from build123d import *

# Parameters (mm, degrees)
F0_R     = 3.5
F1_DEPTH = 7
F2_R     = 3.5
F3_DEPTH = 25
F4_R     = 5.5
F5_DEPTH = 2
F6_W     = 86
F6_H     = 36
F7_DEPTH = 25
F8_R     = 3


with BuildPart() as f1:
    # F0 (on Front) → F1 (new body)
    with BuildSketch(Plane.XZ):
        with BuildLine():
            Line((-57, -60), (57, -60))
            ThreePointArc((57, -60), (59.12132, -59.12132), (60, -57))
            Line((60, -57), (60, 57))
            ThreePointArc((60, 57), (59.12132, 59.12132), (57, 60))
            Line((57, 60), (-57, 60))
            ThreePointArc((-57, 60), (-59.12132, 59.12132), (-60, 57))
            Line((-60, 57), (-60, -57))
            ThreePointArc((-60, -57), (-59.12132, -59.12132), (-57, -60))
        make_face()
        with Locations((-50, -50)):
            Circle(F0_R, mode=Mode.SUBTRACT)
        with Locations((50, -50)):
            Circle(F0_R, mode=Mode.SUBTRACT)
        with Locations((-50, 50)):
            Circle(F0_R, mode=Mode.SUBTRACT)
        with Locations((50, 50)):
            Circle(F0_R, mode=Mode.SUBTRACT)
    extrude(amount=F1_DEPTH)

    # F2 (on face) → F3 (cut)
    with BuildSketch(Plane.XZ.offset(7)):
        with Locations((-32, -10)):
            Circle(F2_R)
        with Locations((-32, -50)):
            Circle(F2_R)
        with Locations((32, -50)):
            Circle(F2_R)
        with Locations((32, -10)):
            Circle(F2_R)
    extrude(amount=-F3_DEPTH, mode=Mode.SUBTRACT)

    # F4 (on face) → F5 (cut)
    with BuildSketch(Plane(origin=(0, 0, 0), x_dir=(-1, 0, 0), z_dir=(0, 1, 0))):
        with Locations((-32, -10)):
            Circle(F4_R)
        with Locations((-32, -50)):
            Circle(F4_R)
        with Locations((32, -50)):
            Circle(F4_R)
        with Locations((32, -10)):
            Circle(F4_R)
    extrude(amount=-F5_DEPTH, mode=Mode.SUBTRACT)

    # F6 (on face) → F7 (cut)
    with BuildSketch(Plane.XZ.offset(7)):
        with Locations((0, 25)):
            Rectangle(F6_W, F6_H)
    extrude(amount=-F7_DEPTH, mode=Mode.SUBTRACT)

    # F8
    f8_edges = [f1.edges().sort_by_distance(p)[0] for p in [
        (-43, -3.5, 43),
        (-43, -3.5, 7),
        (43, -3.5, 43),
        (43, -3.5, 7),
    ]]
    fillet(f8_edges, radius=F8_R)


solid = f1.part
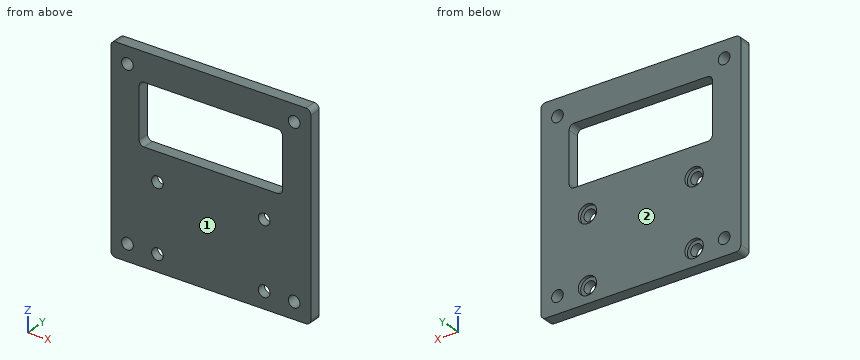
Can you work these out from the model? Positions are in its coordinate system, mm. Face numbers are marked on the shaded views. Coordinates: 2 decimals unless noted, no trailing zeros. Loops run counter-clockwise (first coordinate to the right, second up) from the corner with the lowest first, then second, coordinate; pieces in that order, holes last. Notation, with made-up numbers: M 33,50.5 L 39,50.5 A15 cw 39,66.5 Z; hole C -0.5,15 d5. An arc over 180 degrees is marked long. Return JSON: item names as keys, results as strings. Group by question number.
Item 1: Imagine slicing it at C-C (y = -3.25). Give the number of separate pieces and of enclosed holes in the cut face, and give its area (3 significant figures).
Item 2: Thinking about a two-plate mould opening in Y: for the marked faces 1 and 2, which applies, released by +Y, released by -Y, zero draft, split by the parting line, or undercut?
Item 3: Imagine slicing it at D-D (z = -10). Please give me the cut outline in (x, y).
Item 4: If I drill on L1, parallel to Z at x = -32, y = -5.35; L2, parallel to Z at x = -32, y = -1; L3, parallel to X at y = -2.5, z = 27, over which ranges is the centre line in solid material (lowest first)? Write a range as from..to.
Item 5: Imagine slicing it at A-A (z = 14.5). Please give me the cut outline in (x, y), and give its area (3 significant figures).
Item 6: Imagine slicing it at B-B (x = -50). Please give me the cut outline in (y, z).
Verdict:
{
 "1": {"separate pieces": "1", "enclosed holes": "9", "area": "11,000 mm^2"},
 "2": {"face 1": "released by -Y", "face 2": "released by +Y"},
 "3": {"outline": "M -60,-7 L -35.5,-7 L -35.5,-2 L -37.5,-2 L -37.5,0 L -60,0 Z; M -28.5,-7 L 28.5,-7 L 28.5,-2 L 26.5,-2 L 26.5,0 L -26.5,0 L -26.5,-2 L -28.5,-2 Z; M 35.5,-7 L 60,-7 L 60,0 L 37.5,0 L 37.5,-2 L 35.5,-2 Z"},
 "4": {"L1": "z = -60..-53.5, -46.5..-13.5, -6.5..7, 43..60", "L2": "z = -60..-55.5, -44.5..-15.5, -4.5..7, 43..60", "L3": "x = -60..-43, 43..60"},
 "5": {"outline": "M -60,-7 L -43,-7 L -43,0 L -60,0 Z; M 43,-7 L 60,-7 L 60,0 L 43,0 Z", "area": "238 mm^2"},
 "6": {"outline": "M -7,-60 L 0,-60 L 0,-53.5 L -7,-53.5 Z; M -7,-46.5 L 0,-46.5 L 0,46.5 L -7,46.5 Z; M -7,53.5 L 0,53.5 L 0,60 L -7,60 Z"}
}
